Can you work these out from the model? Positions are in its coordinate system, mm. Face numbers are marked on the shaded views. A direction names the side the tool comes from. Give positions to 0.01 mm unless a question says otherwise; leave off trailing zeros. Loops run counter-clockwise (first coordinate to the right, second up) from the corner with the lowest first, then second, coordinate; pieces in that order, holes last. Notation, with made-up numbers: M 54.25,51.5 L 95.25,51.5 A11 ccw 95.25,67.5 Z; hole C -26,49 d3. An arc over 180 degrees is marked long. Answer as a JSON object with one key per item and string values.
```python
from build123d import *

# Parameters (mm, degrees)
F1_DEPTH = 25.4
F2_DEPTH = 63.5
F3_DEPTH = 15.875


with BuildPart() as f1:
    # F0 (on Front) → F1 (new body, symmetric)
    with BuildSketch(Plane.XZ):
        with BuildLine():
            Line((22.225, 9.525), (41.275, 9.525))
            Line((41.275, 9.525), (41.275, 26.9875))
            ThreePointArc((41.275, 26.9875), (45.92468, 38.21282), (57.15, 42.8625))
            Line((57.15, 42.8625), (60.325, 42.8625))
            Line((60.325, 42.8625), (60.325, 61.9125))
            Line((60.325, 61.9125), (57.15, 61.9125))
            ThreePointArc((57.15, 61.9125), (32.454296, 51.683204), (22.225, 26.9875))
            Line((22.225, 26.9875), (22.225, 9.525))
        make_face()
    extrude(amount=F1_DEPTH, both=True)

    # F0 (on Front) → F2 (join, symmetric)
    with BuildSketch(Plane.XZ):
        Polygon((41.275, -9.525), (41.275, 9.525), (22.225, 9.525), (-41.275, 9.525), (-41.275, -9.525), align=None)
    extrude(amount=F2_DEPTH, both=True)

    # F0 (on Front) → F3 (join)
    with BuildSketch(Plane.XZ):
        with BuildLine():
            Line((-41.275, 9.525), (22.225, 9.525))
            Line((22.225, 9.525), (22.225, 26.9875))
            ThreePointArc((22.225, 26.9875), (32.454296, 51.683204), (57.15, 61.9125))
            add(Edge.make_bspline(
                [(-41.275, 9.525), (-29.119365, 41.789368), (22.899356, 63.857913), (57.15, 61.9125)],
                knots=[0, 0, 0, 0, 111.498569, 111.498569, 111.498569, 111.498569], degree=3))
        make_face()
    extrude(amount=F3_DEPTH)


solid = f1.part
```
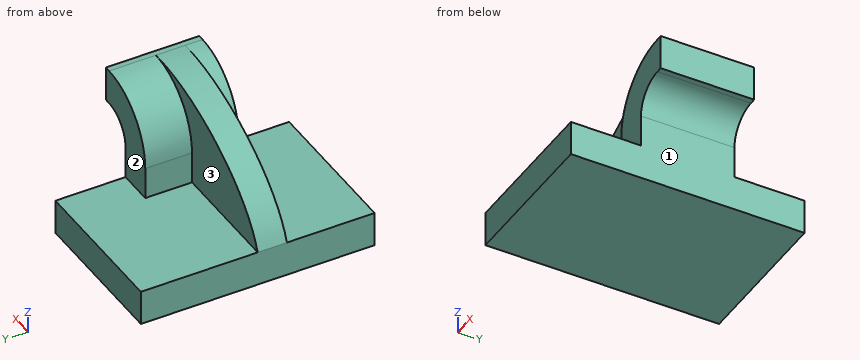
1) Suppose I cut it at B-B, the plane y = -37.5. Write out the boundary of the cut face in (x, z) (3 decimals), and give its area (3 significant figures).
Answer list:
{"outline": "M -41.275,-9.525 L 41.275,-9.525 L 41.275,9.525 L -41.275,9.525 Z", "area": "1,570 mm^2"}
2) For the marked faces 1, 2 and 3, which set-ups out of +Z, -Z, +X, -X, +Y, -Y let a thin tool reach every point of the face, with its end or its side?
Answer list:
{"face 1": "-Z, +X, +Y, -Y", "face 2": "+Z, +X, -X, +Y", "face 3": "+Z, -X, +Y"}
3) Will these pins go through, and if not, where does the flat tip stop? pin 1 Ø5 at (y, z) = (12, -0.5) entering from +X (3 decimals); pin 2 Ø11.5 at (x, z) = (49.5, 47) entering from -Y; pin 3 Ø8.5 at (y, z) = (14, 17.5) entering from -X (3 decimals).
Answer list:
{"pin 1": "x = 41.275", "pin 2": "y = -25.4", "pin 3": "x = 22.225"}
4) Please list where these lines run through material, in increasing order: line 1 along Y through (x, z) = (37, 48); line 2 along X through (y, z) = (15, 23.5) (3 decimals); line 3 along Z through (x, y) = (2.5, 49) (3 decimals). Write a range as from..to.
Answer list:
{"line 1": "-25.4..25.4", "line 2": "22.225..41.275", "line 3": "-9.525..9.525"}
